Autodesk Inventor part; units mm, degrees
ref_plane "YZ Plane" through (0, 0, 0) normal (1, 0, 0) x (0, 1, 0)
ref_plane "XZ Plane" through (0, 0, 0) normal (0, 1, 0) x (-1, 0, 0)
ref_plane "XY Plane" through (0, 0, 0) normal (0, 0, 1) x (1, 0, 0)
sketch "Sketch1" plane through (0, 0, 0) normal (0, 0, 1) x (1, 0, 0)
  line L0 (-42, 0) -> (42, 0)
  line L1 (-30, 0) -> (-30, -20)
  line L2 (-30, -20) -> (-10, -20)
  line L3 (-10, -20) -> (-10, -65)
  line L4 (-10, -65) -> (0, -65)
  line L5 (0, -78) -> (0, 13)
  line L6 (-30, 0) -> (0, 0)
  line L7 (30, 0) -> (30, -20)
  line L8 (30, -20) -> (10, -20)
  line L9 (10, -20) -> (10, -65)
  line L10 (10, -65) -> (0, -65)
  line L11 (30, 0) -> (0, 0)
  line L12 (-30, -10) -> (30, -10) construction
  circle A0 centre (-20, -10) radius 2.4
  circle A1 centre (20, -10) radius 2.4
  dimension "d0" = 10
  dimension "d1" = 20
  dimension "d2" = 65
  dimension "d3" = 30
  dimension "d4" = 10
  dimension "d5" = 4.8
  dimension "d6" = 4.8
  dimension "d7" = 10
  dimension "d8" = 10
extrude "Extrusion1" add sketch "Sketch1" along normal blind 8
sketch "Sketch2" plane through (0, 0, 8) normal (0, 0, 1) x (1, 0, 0)
  circle A0 centre (-20, -10) radius 2.4
  circle A1 centre (20, -10) radius 2.4
  circle A2 centre (-20, -10) radius 5
  circle A3 centre (20, -10) radius 5
  point P0 (0, 0)
  dimension "d11" = 10
  dimension "d12" = 10
extrude "Extrusion2" cut sketch "Sketch2" against normal blind 6
sketch "Sketch3" plane through (0, 0, 8) normal (0, 0, 1) x (1, 0, 0)
  line L0 (0, -78) -> (0, 13)
  circle A0 centre (0, -55) radius 4.15
  circle A1 centre (-20, -10) radius 2.4
  circle A2 centre (0, -55) radius 6.15
  point P0 (0, 0)
  dimension "d15" = 45
  dimension "d16" = 8.3
  dimension "d17" = 2
extrude "Extrusion3" add sketch "Sketch3" along normal blind 10 contours A2 L0 A0 | L0 A0 A2
chamfer "Chamfer1" distance 0.5 angle 45 1 edges at (-4.15, -55, 18)
chamfer "Chamfer2" distance 4 angle 45 1 edges at (-6.15, -55, 8)
fillet "Fillet1" radius 10 4 edges at (10, -65, 4) (-10, -65, 4) (-10, -20, 4) (10, -20, 4)
fillet "Fillet2" radius 2 4 edges at (30, -20, 4) (30, 0, 4) (-30, 0, 4) (-30, -20, 4)
chamfer "Chamfer3" distance 0.5 angle 45 9 edges at (-7.0711, -62.0711, 0) (-10, -42.5, 0) (7.0711, -62.0711, 0) (10, -42.5, 0) (23.9999, -20, 0) (-23.9999, -20, 0) (-30, -10, 0) (0, 0, 0) (30, -10, 0)
chamfer "Chamfer4" distance 2 angle 45 9 edges at (-12.9289, -22.9289, 8) (-23.9999, -20, 8) (-10, -41.6307, 8) (-30, -10, 8) (0, 0, 8) (10, -41.6307, 8) (12.9289, -22.9289, 8) (23.9999, -20, 8) (30, -10, 8)
equation "\"d4\" = 0.5 * d1"
equation "\"d8\" = d7"
equation "\"d12\" = d11"
properties part number "RodHolder_2"
Geometry: final body of the model. Coordinates: model frame, mm. A direction names the side the tool comes from. Give positions to 0.01 mm unless a question says otherwise; leave off trailing zeros. Order: outer loops, then holes, each group sorted by start corner. A loop starts at its lowest first (then second) coordinate and runs counter-clockwise, first axis right, second up. Notation, with made-up numbers: (80, 45.25) -> (136, 45.25) arc R26 ccw to (136, 67.25) -> close; hole circle Ø10 at (28.5, -37.75). An arc over 180 degrees is marked (long way). Answer as a JSON object with one key per item and string values.
Q1. Section D-D (z = 15.5). Output: boundary loops of the cut face in (x, y), plus the area to 3 significant figures.
Entries:
{"outline": "circle Ø12.3 at (0, -55); hole circle Ø8.3 at (0, -55)", "area": "64.7 mm^2"}
Q2. First-contact query: pin 1 (8.5 mm diameter, centred on y = -44.5, z = 3, fed in from -X); pin 2 (6 mm diameter, centred on x = 20, y = -10, fed in from +Z); pin 3 (4 mm diameter, centred on x = 1, y = -53.5, fed in from +Z). Flat tips, straight axial feed; report the tip coordinate or a pass-through.
Entries:
{"pin 1": "stops at x = -10", "pin 2": "stops at z = 2", "pin 3": "stops at z = 8"}
Q3. Access query for faces 4 (the flat face through (-9, -39, 7)), 5 (the flat face through (10, -43, 4)), 6 (the conical face through (29.15, -19.17, 0.14)). Directions: +Z, -Z, +X, -X, +Y, -Y. A direction counts if a zero-diameter tool reaches every point of the face in a straight line with its end or side. Return the directions, or none.
Entries:
{"face 4": "+Z, -X", "face 5": "+Z, -Z, +X, -Y", "face 6": "-Z, +X, -Y"}
Q4. Material intervals for probe 1 along Y at (x, z) = (0, 15); probe 2 along Y at (x, z) = (-20, 0.5); probe 3 along X at (y, z) = (-32, 5.5), sorted ascending.
Entries:
{"probe 1": "y = -61.15 to -59.15, -50.85 to -48.85", "probe 2": "y = -20 to -12.4, -7.6 to 0", "probe 3": "x = -10 to 10"}
Q5. Section C-C (y = -35). Output: boundary loops of the cut face in (x, z), plus the area to 3 significant figures.
Entries:
{"outline": "(-10, 0.5) -> (-9.5, 0) -> (9.5, 0) -> (10, 0.5) -> (10, 6) -> (8, 8) -> (-8, 8) -> (-10, 6) -> close", "area": "156 mm^2"}
Q6. Section A-A (y = -10). Output: boundary loops of the cut face in (x, z), plus the area to 3 significant figures.
Entries:
{"outline": "(-30, 0.5) -> (-29.5, 0) -> (-22.4, 0) -> (-22.4, 2) -> (-25, 2) -> (-25, 8) -> (-28, 8) -> (-30, 6) -> close; (-17.6, 0) -> (17.6, 0) -> (17.6, 2) -> (15, 2) -> (15, 8) -> (-15, 8) -> (-15, 2) -> (-17.6, 2) -> close; (22.4, 0) -> (29.5, 0) -> (30, 0.5) -> (30, 6) -> (28, 8) -> (25, 8) -> (25, 2) -> (22.4, 2) -> close", "area": "337 mm^2"}
Q7. Draft query along X for faces 1 (the flat face through (-24, -19, 7)), 2 (the conical face through (-12.44, -22.61, 6.57)), 3 (the flat face through (17.7, -8.8, 2)). Return one class per face: released by +X, released by -X, zero draft, split by the parting line, or undercut.
Entries:
{"face 1": "zero draft", "face 2": "released by -X", "face 3": "undercut"}
Q8. Section B-B (z = 7). State how many separate pieces and enclosed holes the cut face has, plus the area to 3 significant figures.
Entries:
{"separate pieces": "1", "enclosed holes": "2", "area": "1,750 mm^2"}
